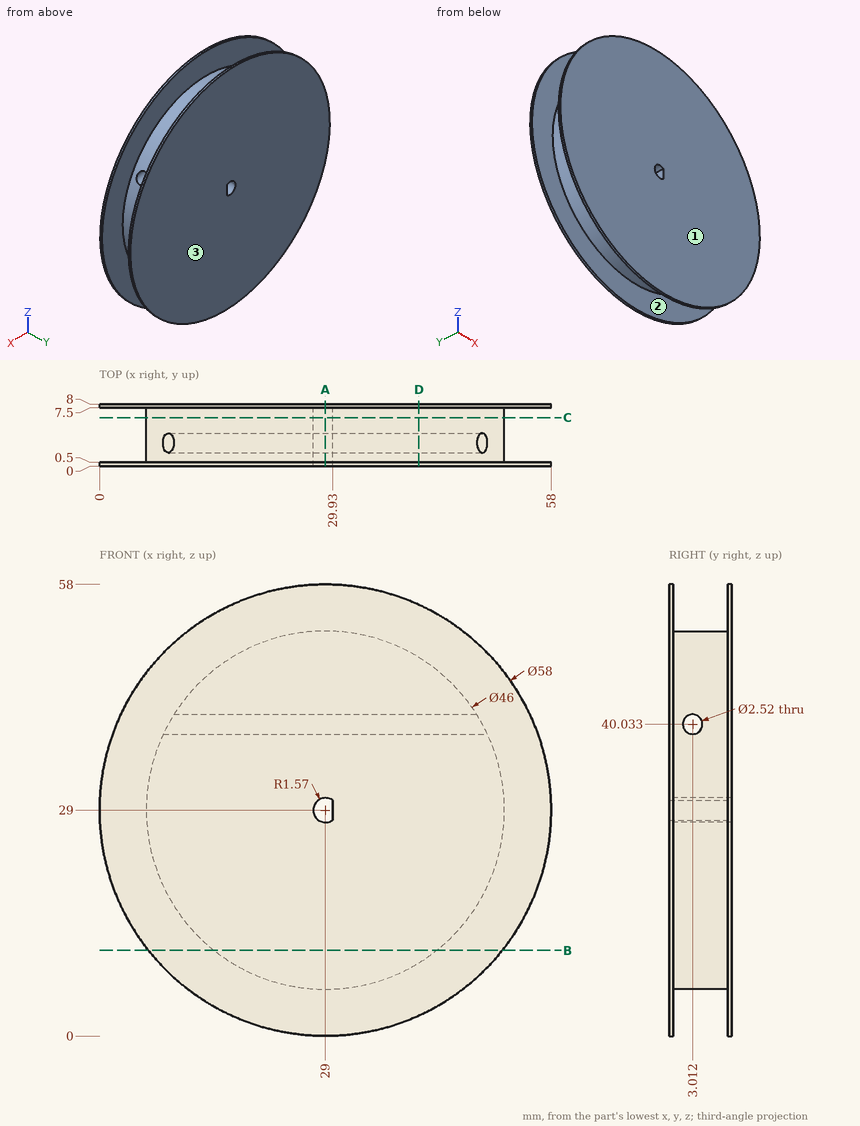
The figure shows three views and two pictorial views of one solid part (mm, origin at its lowest corner). Answer the questions. Give positions to 0.01 mm unless a question says otherwise; leave off trailing zeros. Write each loop counter-clockwise with the first axis right and the second up, starting at its lowest first coordinate (ties: lowest second). Pieces come first, ordered by that corner, then holes. Notation, with made-up numbers: (10, 42) - (67, 42) arc R22 ccw to (67, 68) - close; hole circle Ø11 at (23, 79). An arc over 180 degrees is marked (long way). Use one line per item in the form item = value. Start each with the question number.
1) Flat-ended cylindrical pins translate along their axes: pin 1 Ø2 at (x, y) = (14.5, 3) entering from +Z; pin 2 Ø4 at (x, y) = (31, 3.5) entering from +Z; pin 3 Ø2 at (y, z) = (4.5, 28.5) entering from -X. Find the tip coordinate at first contact, or state that the pin passes through.
2) The mould has two halves that part along Y. Classify the marked faces 1, 2 and 3: pulls with the +Y half, pulls with the -Y half, needs draft (parallel to the pull), parting line crosses it, or undercut.
3) Consider line 1 along Y through (x, z) = (51, 43); line 2 along Z through (x, y) = (29.5, 1) (1 decimal); line 3 along Z through (x, y) = (22.5, 3.75) (1 decimal). Determine where each line is inside the solid, lowest interval first. Write a range as from..to.
4) Find section D-D on x = 41. Determine the outline of the cut face in (y, z).
5) Find section B-B on z = 11. Determine the outline of the cut face in (x, y), plus the area to 3 significant figures.
6) Find section A-A on x = 29. Determine the outline of the cut face in (y, z).
7) Find section C-C on y = 6.25. Determine the outline of the cut face in (x, z) (1 decimal).
Geometry results:
q1.pin_1 = 47.62
q1.pin_2 = 52
q1.pin_3 = 6
q2.face_1 = pulls with the -Y half
q2.face_2 = undercut
q2.face_3 = pulls with the +Y half
q3.line_1 = 0..0.5, 7.5..8
q3.line_2 = 6..27.5, 30.5..52
q3.line_3 = 6.9..39, 41.1..51.1
q4.outline = (0, 2.6) - (0.5, 2.6) - (0.5, 9.38) - (7.5, 9.38) - (7.5, 2.6) - (8, 2.6) - (8, 55.4) - (7.5, 55.4) - (7.5, 48.62) - (0.5, 48.62) - (0.5, 55.4) - (0, 55.4) - close; hole circle Ø2.52 at (3.01, 40.03)
q5.outline = (6.26, 0) - (51.74, 0) - (51.74, 0.5) - (43.32, 0.5) - (43.32, 7.5) - (51.74, 7.5) - (51.74, 8) - (6.26, 8) - (6.26, 7.5) - (14.68, 7.5) - (14.68, 0.5) - (6.26, 0.5) - close
q5.area = 246 mm2
q6.outline = (0, 0) - (0.5, 0) - (0.5, 6) - (7.5, 6) - (7.5, 0) - (8, 0) - (8, 27.43) - (0, 27.43) - close; (0, 30.57) - (8, 30.57) - (8, 58) - (7.5, 58) - (7.5, 52) - (0.5, 52) - (0.5, 58) - (0, 58) - close; hole circle Ø2.52 at (3.01, 40.03)
q7.outline = circle Ø46 at (29, 29); hole (29.9, 27.7) - (29.9, 30.3) arc R1.6 ccw (long way) to start
